Model file for the job. Use its own axes, mm. Face numbers are marked on the shaded views. A direction names the side the tool comes from. Coordinates: 2 decimals unless noted, no trailing zeros. Order: outer loops, then holes, each group sorted by start corner. A loop starts at its lowest first (then second) coordinate and runs counter-clockwise, first axis right, second up.
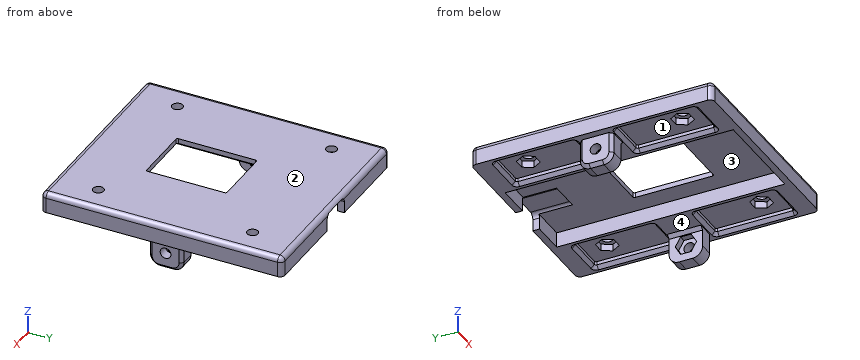
from build123d import *

# Parameters (mm, degrees)
SKETCH082_W     = 62
SKETCH082_H     = 6
PAD030_DEPTH    = 72
FILLET021_R     = 1.5
SKETCH083_W     = 12
SKETCH083_H     = 23.4
POCKET047_DEPTH = 2
FILLET022_R     = 0.5
SKETCH084_W     = 5
SKETCH084_H     = 10
PAD031_DEPTH    = 9
CHAMFER_SIZE    = 1
FILLET023_R     = 3
CHAMFER001_SIZE = 1
SKETCH085_R     = 1.6
POCKET048_DEPTH = 80
POCKET049_DEPTH = 51.6
POCKET050_DEPTH = 12
SKETCH088_W     = 18
SKETCH088_H     = 24
POCKET051_DEPTH = 16
FILLET024_R     = 0.5
SKETCH089_R     = 1.6
POCKET052_DEPTH = 10
POCKET053_DEPTH = 2
SKETCH091_W     = 30
SKETCH091_H     = 68
POCKET054_DEPTH = 4.5
CHAMFER002_SIZE = 1


with BuildPart() as part:
    # Sketch082 → Pad030 (new body)
    with BuildSketch(Plane.XZ.offset(-36)):
        with Locations((0, 25.5)):
            Rectangle(SKETCH082_W, SKETCH082_H)
    extrude(amount=PAD030_DEPTH)

    # Fillet021
    fillet021_edges = [part.edges().sort_by_distance(p)[0] for p in [
        (31, 0, 28.5),
        (-31, 0, 28.5),
        (0, 36, 28.5),
        (0, -36, 28.5),
        (31, -36, 25.5),
        (-31, -36, 25.5),
        (31, 36, 25.5),
        (-31, 36, 25.5),
    ]]
    fillet(fillet021_edges, radius=FILLET021_R)

    # Sketch083 (on Face1 of Fillet021) → Pocket047 (cut)
    with BuildSketch(Plane(origin=(0, 0, 22.5), x_dir=(1, 0, 0), z_dir=(0, 0, -1))):
        with Locations((23, 18)):
            Rectangle(SKETCH083_W, SKETCH083_H)
        with Locations((23, -18)):
            Rectangle(SKETCH083_W, SKETCH083_H)
        with Locations((-23, 18)):
            Rectangle(SKETCH083_W, SKETCH083_H)
        with Locations((-23, -18)):
            Rectangle(SKETCH083_W, SKETCH083_H)
    extrude(amount=-POCKET047_DEPTH, mode=Mode.SUBTRACT)

    # Fillet022
    fillet022_edges = [part.edges().sort_by_distance(p)[0] for p in [
        (17, 6.3, 23.5),
        (17, -6.3, 23.5),
        (29, -6.3, 23.5),
        (17, 29.7, 23.5),
        (29, 29.7, 23.5),
        (29, 6.3, 23.5),
        (17, -29.7, 23.5),
        (29, -29.7, 23.5),
        (-17, -29.7, 23.5),
        (-29, -29.7, 23.5),
        (-29, -6.3, 23.5),
        (-17, -6.3, 23.5),
        (-29, 6.3, 23.5),
        (-17, 6.3, 23.5),
        (-17, 29.7, 23.5),
        (-29, 29.7, 23.5),
    ]]
    fillet(fillet022_edges, radius=FILLET022_R)

    # Sketch084 (on Face1 of Fillet022) → Pad031 (join)
    with BuildSketch(Plane(origin=(0, 0, 22.5), x_dir=(1, 0, 0), z_dir=(0, 0, -1))):
        with Locations((26.3, 0)):
            Rectangle(SKETCH084_W, SKETCH084_H)
        with Locations((-26.3, 0)):
            Rectangle(SKETCH084_W, SKETCH084_H)
    extrude(amount=PAD031_DEPTH)

    # Chamfer
    chamfer_edges = [part.edges().sort_by_distance(p)[0] for p in [
        (23.8, 0, 22.5),
        (-23.8, 0, 22.5),
    ]]
    chamfer(chamfer_edges, length=CHAMFER_SIZE)

    # Fillet023
    fillet023_edges = [part.edges().sort_by_distance(p)[0] for p in [
        (26.3, -5, 13.5),
        (26.3, 5, 13.5),
        (-26.3, -5, 13.5),
        (-26.3, 5, 13.5),
    ]]
    fillet(fillet023_edges, radius=FILLET023_R)

    # Chamfer001
    chamfer001_edges = [part.edges().sort_by_distance(p)[0] for p in [
        (28.8, 0, 13.5),
        (-28.8, 0, 13.5),
    ]]
    chamfer(chamfer001_edges, length=CHAMFER001_SIZE)

    # Sketch085 (on Face55 of Chamfer001) → Pocket048 (cut)
    with BuildSketch(Plane(origin=(-28.8, 0, 0), x_dir=(0, 0, -1), z_dir=(-1, 0, 0))):
        with Locations((-18.5, 0)):
            Circle(SKETCH085_R)
    extrude(amount=-POCKET048_DEPTH, mode=Mode.SUBTRACT)

    # Sketch086 (on Face4 of Pocket048) → Pocket049 (cut)
    with BuildSketch(Plane(origin=(25.8, 0, 0), x_dir=(0, 0, -1), z_dir=(-1, 0, 0))):
        Polygon((-18.5, 3.175426), (-21.25, 1.587713), (-21.25, -1.587713), (-18.5, -3.175426), (-15.75, -1.587713), (-15.75, 1.587713), align=None)
    extrude(amount=POCKET049_DEPTH, mode=Mode.SUBTRACT)

    # Sketch087 (on Face22 of Pocket049) → Pocket050 (cut)
    with BuildSketch(Plane(origin=(0, 36, 0), x_dir=(1, 0, 0), z_dir=(0, 1, 0))):
        with BuildLine():
            Line((-5, -22.5), (-5, -26))
            ThreePointArc((-5, -26), (-4.56066, -27.06066), (-3.5, -27.5))
            Line((-3.5, -27.5), (3.5, -27.5))
            ThreePointArc((3.5, -27.5), (4.56066, -27.06066), (5, -26))
            Line((5, -26), (5, -22.5))
            Line((-5, -22.5), (5, -22.5))
        make_face()
    extrude(amount=-POCKET050_DEPTH, mode=Mode.SUBTRACT)

    # Sketch088 (on Face95 of Pocket050) → Pocket051 (cut)
    with BuildSketch(Plane(origin=(0, 0, 28.5), x_dir=(-1, 0, 0), z_dir=(0, 0, 1))):
        with Locations((0, 4)):
            Rectangle(SKETCH088_W, SKETCH088_H)
    extrude(amount=-POCKET051_DEPTH, mode=Mode.SUBTRACT)

    # Fillet024
    fillet024_edges = [part.edges().sort_by_distance(p)[0] for p in [
        (9, 8, 25.5),
        (9, -16, 25.5),
        (-9, -16, 25.5),
        (-9, 8, 25.5),
    ]]
    fillet(fillet024_edges, radius=FILLET024_R)

    # Sketch089 (on Face66 of Fillet024) → Pocket052 (cut)
    with BuildSketch(Plane(origin=(0, 0, 28.5), x_dir=(-1, 0, 0), z_dir=(0, 0, 1))):
        with Locations((23, 23)):
            Circle(SKETCH089_R)
        with Locations((-23, 23)):
            Circle(SKETCH089_R)
        with Locations((-23, -23)):
            Circle(SKETCH089_R)
        with Locations((23, -23)):
            Circle(SKETCH089_R)
    extrude(amount=-POCKET052_DEPTH, mode=Mode.SUBTRACT)

    # Sketch090 (on Face95 of Pocket052) → Pocket053 (cut)
    with BuildSketch(Plane(origin=(0, 0, 24.5), x_dir=(1, 0, 0), z_dir=(0, 0, -1))):
        Polygon((-21.412287, 25.75), (-24.587713, 25.75), (-26.175426, 23), (-24.587713, 20.25), (-21.412287, 20.25), (-19.824574, 23), align=None)
        Polygon((21.412287, 25.75), (19.824574, 23), (21.412287, 20.25), (24.587713, 20.25), (26.175426, 23), (24.587713, 25.75), align=None)
        Polygon((-19.824574, -23), (-21.412287, -20.25), (-24.587713, -20.25), (-26.175426, -23), (-24.587713, -25.75), (-21.412287, -25.75), align=None)
        Polygon((26.175426, -23), (24.587713, -20.25), (21.412287, -20.25), (19.824574, -23), (21.412287, -25.75), (24.587713, -25.75), align=None)
    extrude(amount=-POCKET053_DEPTH, mode=Mode.SUBTRACT)

    # Sketch091 (on Face1 of Pocket053) → Pocket054 (cut)
    with BuildSketch(Plane(origin=(0, 0, 22.5), x_dir=(1, 0, 0), z_dir=(0, 0, -1))):
        Rectangle(SKETCH091_W, SKETCH091_H)
    extrude(amount=-POCKET054_DEPTH, mode=Mode.SUBTRACT)

    # Chamfer002
    chamfer002_edges = [part.edges().sort_by_distance(p)[0] for p in [
        (-23, -6.3, 22.5),
        (-23, 6.3, 22.5),
        (23, -6.3, 22.5),
        (23, 6.3, 22.5),
    ]]
    chamfer(chamfer002_edges, length=CHAMFER002_SIZE)


with BuildPart() as part_1:
    # Body006 placement: moved
    add(part.part.moved(Location((0, 0, 1))))


solid = part_1.part
Q1. Cut at A-A, the plane y = -10. List the corners of the cut face in (x, z), plus the area to 3 significant figures.
Established:
outline: (-31, 23.5) - (-30, 23.5) - (-29, 24.5) - (-29, 25.5) - (-17, 25.5) - (-17, 24.5) - (-16, 23.5) - (-15, 23.5) - (-15, 28) - (-9, 28) - (-9, 29.5) - (-29.5, 29.5) arc R1.5 ccw to (-31, 28) - close; (9, 28) - (15, 28) - (15, 23.5) - (16, 23.5) - (17, 24.5) - (17, 25.5) - (29, 25.5) - (29, 24.5) - (30, 23.5) - (31, 23.5) - (31, 28) arc R1.5 ccw to (29.5, 29.5) - (9, 29.5) - close
area: 159 mm2
Q2. Probe line 1 (X direction, y = 23, z = 28.2); line 2 (X direction, y = -25, z = 24.75); line 3 (X direction, y = -23, z = 27.9). List the from-to ranges inside material, lowest first.
Established:
line 1: x = -30.99 to -24.6, -21.4 to 21.4, 24.6 to 30.99
line 2: x = -31 to -29, -17 to -15, 15 to 17, 29 to 31
line 3: x = -31 to -24.6, -21.4 to -15, 15 to 21.4, 24.6 to 31
Q3. Which spindle directions (+Z, -Z, +X, -X, +Y, -Y) get a long thin tool onto all of the face, cutting with end or side? Do the marked faces 1 and 2. Say none if no direction does.
Established:
face 1: -Z
face 2: +Z, +X, -X, +Y, -Y
Q4. Mould opens along Y. For the marked faces 3 and 4 say: pulls with the +Y half, pulls with the -Y half, needs draft (parallel to the pull), parting line crosses it, or undercut.
Established:
face 3: undercut
face 4: needs draft
Q5. Drop flat-ended pins along their axis: P1, Ø9.5, axis at x = 26, y = -15.5, coming from the -Z side; P2, Ø1.6, axis at x = 2, z = 28.5, coming from the +Y side; P3, Ø1.9, axis at y = 0, z = 19.5, coming from the +X side; P4, Ø1.6, axis at y = 0.5, z = 29, coming from the +X side. Give the stop position or say it passes through.
Established:
P1: stops at z = 23.5
P2: stops at y = 35.91
P3: passes through
P4: stops at x = 30.99
Q6. Cut at C-C, the plane y = 0. Count the separate pieces of the cut face and the enclosed holes in it, plus the area to 3 significant figures.
Established:
separate pieces: 4
enclosed holes: 0
area: 258 mm2
Q7. Cut at B-B, the plane x = -13. List the corners of the cut face in (y, z), plus the area to 3 significant figures.
Established:
outline: (-36, 23.5) - (-34, 23.5) - (-34, 28) - (34, 28) - (34, 23.5) - (36, 23.5) - (36, 28) arc R1.5 ccw to (34.5, 29.5) - (-34.5, 29.5) arc R1.5 ccw to (-36, 28) - close
area: 125 mm2
